CAD build for the part. Positions are in the model's coordinates, mm. A direction names the side the tool comes from. Coordinates: 2 decimals unless noted, no trailing zeros. Order: outer loops, then holes, each group sorted by start corner. A loop starts at its lowest first (then second) coordinate and runs counter-clockwise, first axis right, second up. Notation, with made-up numbers: (83, -16.5) - (134, -16.5) arc R15 ccw to (134, 7.5) - close; hole circle Ø7 at (-39.75, -38). An arc over 180 degrees is marked (long way). Use one line per item in the form item = value.
```python
from build123d import *

# Parameters (mm, degrees)
F1_DEPTH     = 3
F0_W         = 3.4999997824
F0_H         = 12.75
F2_DEPTH     = 22
F0_W_2       = 10.8
F0_H_2       = 3.4999997824
F3_DEPTH     = 5
F4_SIZE      = 5
F5_DEPTH     = 17.9
F6_T4_DEPTH  = 29.2168296621
F6_T9_DEPTH  = 29.2168296621
F7_W         = 3.4999997824
F7_H         = 4.4000236183
F8_DEPTH     = 8.1
F9_W         = 3.4999997824
F9_H         = 5.7981096033
F9_H_2       = 0.0001660025
F9_W_2       = 14.2999671862
F10_DEPTH    = 1.59
F11_DEPTH    = 5
F13_DEPTH    = 2.02
F14_T4_DEPTH = 36.5168298797


# Not quite as in the source:
# - a fillet or chamfer that OpenCascade refuses, or shapes differently, is made with other operations: its cross-section is extruded or revolved along the edge and cut away or added
# - ends of sketch curves that miss each other by under 0.0002 mm in the source are joined


with BuildPart() as f1:
    # F0 (on Top) → F1 (new body)
    with BuildSketch(Plane.XY):
        Polygon((5.4, 0), (5.4, 12.75), (-5.4, 12.75), (-5.4, 0), (-5.4, -12.75), (5.4, -12.75), align=None)
    extrude(amount=F1_DEPTH)

    # F0 (on Top) → F2 (join)
    with BuildSketch(Plane.XY):
        with Locations((-7.1499998912, 6.375)):
            Rectangle(F0_W, F0_H)
        with Locations((7.1499998912, 6.375)):
            Rectangle(F0_W, F0_H)
        Polygon((-5.4, -12.75), (-5.4, 0), (-8.8999997824, 0), (-8.8999997824, -16.2499997824), (-5.4, -16.2499997824), align=None)
        Polygon((8.8999997824, 0), (5.4, 0), (5.4, -12.75), (5.4, -16.2499997824), (8.8999997824, -16.2499997824), align=None)
    extrude(amount=F2_DEPTH)

    # F0 (on Top) → F3 (join)
    with BuildSketch(Plane.XY):
        with Locations((0, 14.4999998912)):
            Rectangle(F0_W_2, F0_H_2)
        with Locations((-7.1499998912, 14.4999998912)):
            Rectangle(F0_W, F0_H_2)
        with Locations((7.1499998912, 14.4999998912)):
            Rectangle(F0_W, F0_H_2)
    extrude(amount=F3_DEPTH)

    # F4
    f4_edges = [f1.edges().sort_by_distance(p)[0] for p in [
        (-7.15, -16.25, 22),
        (7.15, -16.25, 22),
    ]]
    chamfer(f4_edges, length=F4_SIZE)

    # F0 (on Top) → F5 (join)
    with BuildSketch(Plane.XY):
        with Locations((-7.1499998912, 14.4999998912)):
            Rectangle(F0_W, F0_H_2)
        with Locations((7.1499998912, 14.4999998912)):
            Rectangle(F0_W, F0_H_2)
    extrude(amount=F5_DEPTH)

    # F6: chamfer of 5 on 2 edges, made by hand


with BuildPart() as f6_tool2:
    # F6_s3 → F6_t4 (new body)
    with BuildSketch(Plane.YZ.offset(21.7584147223)):
        Polygon((7.75, 22), (12.75, 17), (12.75, 22), align=None)
    extrude(amount=-F6_T4_DEPTH)

    split(bisect_by=Plane.XY.offset(17.9), keep=Keep.TOP)


with BuildPart() as f1_1:
    add(f1.part)

    # F6_t1: cut F6_tool2
    add(f6_tool2.part, mode=Mode.SUBTRACT)


with BuildPart() as f6_tool7:
    # F6_s8 → F6_t9 (new body)
    with BuildSketch(Plane.YZ.offset(7.4584149398)):
        Polygon((12.75, 17), (7.75, 22), (12.75, 22), align=None)
    extrude(amount=-F6_T9_DEPTH)

    split(bisect_by=Plane.XY.offset(17.9), keep=Keep.TOP)


with BuildPart() as f1_2:
    add(f1_1.part)

    # F6_t6: cut F6_tool7
    add(f6_tool7.part, mode=Mode.SUBTRACT)

    # F7 (on face) → F8 (join)
    with BuildSketch(Plane.XY.offset(17.9)):
        with Locations((7.1499998912, 14.0500118092)):
            Rectangle(F7_W, F7_H)
        Polygon((-8.9000016451, 11.85), (5.4, 11.85), (5.4, 16.2499997824), (-8.9000016451, 16.2500236183), align=None)
    extrude(amount=-F8_DEPTH)

    # F9 (on face) → F10 (join)
    with BuildSketch(Plane(origin=(0, 14.875, 14.875), x_dir=(-1, 0, 0), z_dir=(0, 0.7071067812, 0.7071067812))):
        with Locations((-7.1499998912, 7.1772168303)):
            Rectangle(F9_W, F9_H)
        with Locations((-7.1499998912, 4.2780790274)):
            Rectangle(F9_W, F9_H_2)
        with Locations((1.7499835931, 7.1772168303)):
            Rectangle(F9_W_2, F9_H)
    extrude(amount=-F10_DEPTH)

    # F0 (on Top) → F11 (join)
    with BuildSketch(Plane.XY):
        with Locations((0, -14.4999998912)):
            Rectangle(F0_W_2, F0_H_2)
    extrude(amount=F11_DEPTH)

    # F12 (on face) → F13 (join)
    with BuildSketch(Plane.XY.offset(22)):
        Polygon((5.4, -11.2499997824), (5.4, 7.75), (-8.8998991996, 7.75), (-8.8998991996, -11.2499557436), align=None)
    extrude(amount=-F13_DEPTH)

    # F14: chamfer of 5 on 1 edges, made by hand


with BuildPart() as f14_tool2:
    # F14_s3 → F14_t4 (new body)
    with BuildSketch(Plane(origin=(-18.2583802936, 5.62297e-05, 0), x_dir=(0, 0, 1), z_dir=(1, -3.0797e-06, 0))):
        Polygon((19.98, 6.2499831522), (24.98, 11.2499831522), (19.98, 11.2499831522), align=None)
    extrude(amount=F14_T4_DEPTH)

    split(bisect_by=Plane.YZ.offset(5.4), keep=Keep.BOTTOM)

    split(bisect_by=Plane.YZ.offset(-5.4), keep=Keep.TOP)


with BuildPart() as f1_3:
    add(f1_2.part)

    # F14_t1: cut F14_tool2
    add(f14_tool2.part, mode=Mode.SUBTRACT)


solid = f1_3.part
```
Item 1: Drop flat-ended pins along their axis: pin 1 (4 mm diameter, centred on x = 1, z = 13.5, fed in from -Y); pin 2 (3 mm diameter, centred on x = -2, y = -14.5, fed in from +Z); pin 3 (5 mm diameter, centred on x = -3, y = 13.5, fed in from +Z). Give the stop position or say it passes through.
Derived:
pin_1 = 11.85
pin_2 = 5
pin_3 = 18.75
Item 2: Cut at A-A, the plane y = 6. Write the cut outline in (x, z), plus the area to 3 significant figures.
Derived:
outline = (-8.9, 0) - (8.9, 0) - (8.9, 22) - (-8.9, 22) - close; hole (-5.4, 3) - (5.4, 3) - (5.4, 19.98) - (-5.4, 19.98) - close
area = 208 mm²
Item 3: Cut at B-B, the plane z = 6. Write the cut outline in (x, y).
Derived:
outline = (-8.9, -16.25) - (-5.4, -16.25) - (-5.4, 16.25) - (-8.9, 16.25) - close; (5.4, -16.25) - (8.9, -16.25) - (8.9, 16.25) - (5.4, 16.25) - close
Item 4: Cut at C-C, the plane x = 0. Write the cut outline in (y, z), plus the area to 3 significant figures.
Derived:
outline = (-16.25, 0) - (16.25, 0) - (16.25, 5) - (12.75, 5) - (12.75, 3) - (-12.75, 3) - (-12.75, 5) - (-16.25, 5) - close; (-8.27, 22) - (-6.25, 19.98) - (7.52, 19.98) - (10.73, 16.78) - (11.85, 17.9) - (7.75, 22) - close; (11.85, 9.8) - (16.25, 9.8) - (16.25, 17.9) - (11.85, 17.9) - close
area = 185 mm²
Item 5: 3-axis set-ups, long thin cutter, end or side, ignore diameter. For faces 1 (the face through (0, 15, 5)), 2 (the face through (0, 12.75, 4)), 3 (the face through (0, -14, 5)): which of +Z, -Z, +X, -X, +Y, -Y reach the whole face in a straight line?
Derived:
face_1 = +Y, -Y
face_2 = none
face_3 = +Z, +Y, -Y
Item 6: Cut at D-D, the plane y = -10. Write the cut outline in (x, z), plus the area to 3 significant figures.
Derived:
outline = (-8.9, 0) - (8.9, 0) - (8.9, 22) - (5.4, 22) - (5.4, 3) - (-5.4, 3) - (-5.4, 22) - (-8.9, 22) - close
area = 186 mm²
Item 7: Drill centre lines: line 1 (Z direction, x = 4.75, y = 13.5); line 2 (X direction, y = 7, z = 18); line 3 (Z direction, x = -3.5, y = 4.5). Where is each one in solid material? Low to high. Write a range as [from, to].
Derived:
line_1 = [0, 5], [9.8, 17.9]
line_2 = [-8.9, -5.4], [5.4, 8.9]
line_3 = [0, 3], [19.98, 22]
Item 8: Two-plate mould, pull along Y, no slides. Class faces 4 (the face through (-0.1, -16.25, 4.6)), 5 (the face through (0, 1, 19.98)), 6 (the face through (0, -12.75, 4)), 7 (the face through (0.12, 9.77, 19.98)): +Y half, -Y half, draft (parallel to the pull), parting line (faces both ways), or undercut.
Derived:
face_4 = -Y half
face_5 = draft
face_6 = undercut
face_7 = +Y half
